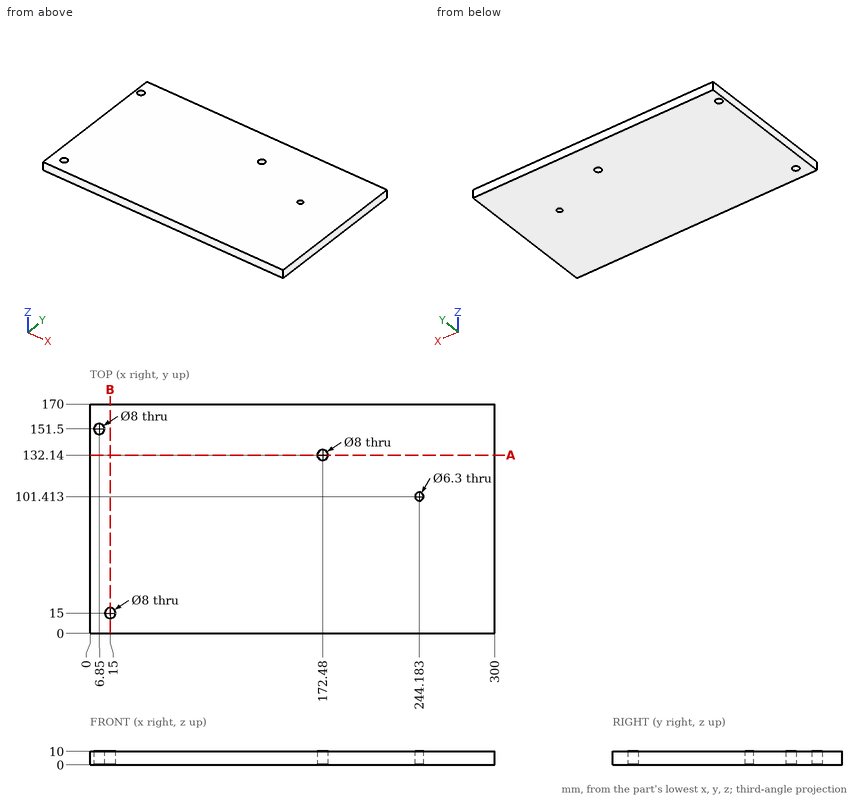
Geometry: see drawing. Coordinates: mm, zero at the bounding-box minimum. Coordinates: 2 decimals unless noted, no trailing zeros. Loops run counter-clockwise (first coordinate to the right, second up) from the corner with the lowest first, then second, coordinate; pieces in that order, holes last. Notation, with made-up numbers: (-31.75, -11.75) - (25.25, -11.75) arc R22 ccw to (25.25, 12.25) - close; hole circle Ø6 at (79, 4). An arc over 180 degrees is marked (long way). Answer as CSV lines item,"result".
1. Ray query, line 1 (Y direction, x = 172.48, z = 6.75); line 2 (Y direction, x = 176, z = 7.5); line 3 (X direction, y = 100, z = 0.5). Return the intervals inside material, ascending.
Established:
line 1,"y = 0 to 128.14, 136.14 to 170"
line 2,"y = 0 to 130.24, 134.04 to 170"
line 3,"x = 0 to 241.37, 247 to 300"
2. Section B-B (x = 15). Return loops of the section in (y, z).
Established:
outline,"(0, 0) - (11, 0) - (11, 10) - (0, 10) - close; (19, 0) - (170, 0) - (170, 10) - (19, 10) - close"
3. Contact query for flat-ended pins moving along their axis: pin 1 (8 mm diameter, centred on x = 117.5, y = 98, fed in from -Z); pin 2 (6.5 mm diameter, centred on x = 172.48, y = 132.14, fed in from -Z). Output: stop coordinate, or through.
Established:
pin 1,"stops at z = 0"
pin 2,"passes through"
4. Section A-A (y = 132.14). Return loops of the section in (x, z), then the cut area to 3 significant figures.
Established:
outline,"(0, 0) - (168.48, 0) - (168.48, 10) - (0, 10) - close; (176.48, 0) - (300, 0) - (300, 10) - (176.48, 10) - close"
area,"2,920 mm2"
